from build123d import *

# Parameters (mm, degrees)
SKETCH015_R      = 1.2
EXTRUDE011_DEPTH = 10
SKETCH006_W      = 11.2
SKETCH006_H      = 38
EXTRUDE001_DEPTH = 1
SKETCH007_R      = 1
SKETCH007_W      = 6.4
SKETCH007_H      = 15
SKETCH007_W_2    = 2
SKETCH007_W_3    = 14.5
SKETCH007_H_2    = 2
SKETCH007_W_4    = 22.95
EXTRUDE005_DEPTH = 2.6
SKETCH005_W      = 51.25
SKETCH005_H      = 53
EXTRUDE_DEPTH    = 2
SKETCH013_R      = 1.65
EXTRUDE009_DEPTH = 5
SKETCH012_R      = 3
EXTRUDE008_DEPTH = 5


with BuildPart() as basecut:
    # Sketch015 → Extrude011 (new body)
    with BuildSketch(Plane.XY):
        with Locations((22.75, 50)):
            Circle(SKETCH015_R)
        with Locations((22.75, 3.25)):
            Circle(SKETCH015_R)
    extrude(amount=EXTRUDE011_DEPTH)


with BuildPart() as base002:
    # Sketch006 → Extrude001 (new body)
    with BuildSketch(Plane.XY.offset(2)):
        with Locations((37.6, 27)):
            Rectangle(SKETCH006_W, SKETCH006_H)
    extrude(amount=EXTRUDE001_DEPTH)


with BuildPart() as base003:
    # Sketch007 → Extrude005 (new body)
    with BuildSketch(Plane.XY.offset(2)):
        with Locations((28.675, 48.25)):
            Circle(SKETCH007_R)
        with Locations((46.475, 48.25)):
            Circle(SKETCH007_R)
        with Locations((28.675, 2.55)):
            Circle(SKETCH007_R)
        with Locations((46.475, 2.55)):
            Circle(SKETCH007_R)
        Polygon((3.25, 0), (5.25, 0), (5.25, 5.25), (6.75, 5.25), (6.75, 7.25), (3.25, 7.25), align=None)
        Polygon((17.75, 0), (15.75, 0), (15.75, 1.1), (15.3, 1.1), (15.3, 1.9), (15.75, 1.9), (15.75, 5.25), (14.25, 5.25), (14.25, 7.25), (17.75, 7.25), align=None)
        with Locations((22.7, 27.5)):
            Rectangle(SKETCH007_W, SKETCH007_H)
        with Locations((1, 27.5)):
            Rectangle(SKETCH007_W_2, SKETCH007_H)
        with Locations((10.5, 52)):
            Rectangle(SKETCH007_W_3, SKETCH007_H_2)
        with Locations((50.25, 27.5)):
            Rectangle(SKETCH007_W_2, SKETCH007_H)
        with Locations((37.575, 52)):
            Rectangle(SKETCH007_W_4, SKETCH007_H_2)
    extrude(amount=EXTRUDE005_DEPTH)


with BuildPart() as base004:
    # Sketch005 → Extrude (new body)
    with BuildSketch(Plane.XY):
        with Locations((25.625, 26.5)):
            Rectangle(SKETCH005_W, SKETCH005_H)
    extrude(amount=EXTRUDE_DEPTH)

    # Fusion002: union base002, base003
    add(base002.part)
    add(base003.part)


with BuildPart() as extrude009:
    # Sketch013 → Extrude009 (new body)
    with BuildSketch(Plane.XY.offset(10.25)):
        with Locations((22.75, 50)):
            Circle(SKETCH013_R)
        with Locations((22.75, 3.25)):
            Circle(SKETCH013_R)
    extrude(amount=EXTRUDE009_DEPTH)


with BuildPart() as extrude009_1:
    # Extrude009 placement: moved
    add(extrude009.part.moved(Location((0, 0, -8.25))))


with BuildPart() as bottom001:
    # Sketch012 → Extrude008 (new body)
    with BuildSketch(Plane.XY.offset(10.25)):
        with Locations((22.75, 50)):
            Circle(SKETCH012_R)
        with Locations((22.75, 3.25)):
            Circle(SKETCH012_R)
    extrude(amount=EXTRUDE008_DEPTH)


with BuildPart() as bottom001_1:
    # Extrude008 placement: moved
    add(bottom001.part.moved(Location((0, 0, -8.25))))

    # Cut002: cut Extrude009
    add(extrude009_1.part, mode=Mode.SUBTRACT)

    # Fusion003: union base004
    add(base004.part)

    # Cut004: cut baseCut
    add(basecut.part, mode=Mode.SUBTRACT)


solid = bottom001_1.part
Source: CAD feature listing. Evaluate the final solid. Frame: model axes, mm. A direction names the side the tool comes from. Give positions to 0.01 mm unless a question says otherwise; leave off trailing zeros. Write each loop counter-clockwise with the first axis right and the second up, starting at its lowest first coordinate (ties: lowest second). Pieces come first, ordered by that corner, then holes. Notation, with made-up numbers: (56.25, 85) -> (94.25, 85) arc R16 cw to (94.25, 96) -> close; hole circle Ø11 at (-32, -31). An arc over 180 degrees is marked (long way). Return JSON: item names as keys, results as strings. Group by question number.
1. Material intervals for line 1 (Y direction, x = 20, z = 2.5); line 2 (Y direction, x = 22.75, z = 0.75); line 3 (Y direction, x = 22.75, z = 5.6), sorted ascending. Write a range as from..to.
2. Section B-B, the plane y = 16. Output: boundary loops of the cut face in (x, z).
3. Access query for faces 1 (the face through (23, 35, 3)), 2 (the face through (1, 35, 3)), 3 (the face through (37, 52, 4.6)), 4 (the face through (14.25, 6, 3)), 5 (the face through (17.75, 52, 3)). Directions: +Z, -Z, +X, -X, +Y, -Y. A direction counts if a zero-diameter tool reaches every point of the face in a straight line with its end or side. Return the directions, or none.
4. Mould query, pull axis X, two halves, no side actions, for faces 6 (the face through (19.753, 3.382, 4.465)), 7 (the face through (23, 28, 4.6)), 8 (the face through (3.25, 4, 3)). Classes: +X half, -X half, draft (parallel to the pull), parting line (faces both ways), or undercut.
5. Section D-D, the plane x = 37. Output: boundary loops of the cut face in (y, z).
6. Section A-A, the plane y = 50. Output: boundary loops of the cut face in (x, z).
7. Section C-C, the plane z = 5.75. Output: boundary loops of the cut face in (x, y), then the cut area to 3 significant figures.
8. Pin query (flat end, axial travel): pin 1 Ø1.3 at (y, z) = (3, 3.5) entering from -X; pin 2 Ø3 at (x, y) = (23.5, 25) entering from +Z; pin 3 Ø3.5 at (x, y) = (38, 26) entering from +Z. Return the tip coordinate at first contact, or that it passes through.
Determined:
{
 "1": {"line 1": "y = 2.05..4.45, 20..35, 48.8..51.2", "line 2": "y = 0..2.05, 4.45..48.8, 51.2..53", "line 3": "y = 0.25..1.6, 4.9..6.25, 47..48.35, 51.65..53"},
 "2": {"outline": "(0, 0) -> (51.25, 0) -> (51.25, 2) -> (43.2, 2) -> (43.2, 3) -> (32, 3) -> (32, 2) -> (0, 2) -> close"},
 "3": {"face 1": "+Z, -X", "face 2": "+Z, -X, +Y", "face 3": "+Z, +X, +Y, -Y", "face 4": "+Z, -Y", "face 5": "+Z, +Y, -Y"},
 "4": {"face 6": "undercut", "face 7": "draft", "face 8": "-X half"},
 "5": {"outline": "(0, 0) -> (53, 0) -> (53, 4.6) -> (51, 4.6) -> (51, 2) -> (46, 2) -> (46, 3) -> (8, 3) -> (8, 2) -> (0, 2) -> close"},
 "6": {"outline": "(0, 0) -> (21.55, 0) -> (21.55, 2) -> (21.1, 2) -> (21.1, 7) -> (19.75, 7) -> (19.75, 2) -> (0, 2) -> close; (23.95, 0) -> (51.25, 0) -> (51.25, 2) -> (25.75, 2) -> (25.75, 7) -> (24.4, 7) -> (24.4, 2) -> (23.95, 2) -> close"},
 "7": {"outline": "circle Ø6 at (22.75, 3.25); circle Ø6 at (22.75, 50); hole circle Ø3.3 at (22.75, 3.25); hole circle Ø3.3 at (22.75, 50)", "area": "39.4 mm2"},
 "8": {"pin 1": "stops at x = 3.25", "pin 2": "stops at z = 4.6", "pin 3": "stops at z = 3"}
}
